For this review, take the finished solid that the model builds, in its own axes (mm). Face numbers are marked on the shaded views. A direction names the side the tool comes from. Give positions to 0.01 mm unless a question says otherwise; leave off trailing zeros. Loops run counter-clockwise (first coordinate to the right, second up) from the corner with the lowest first, then second, coordinate; pieces in that order, holes last.
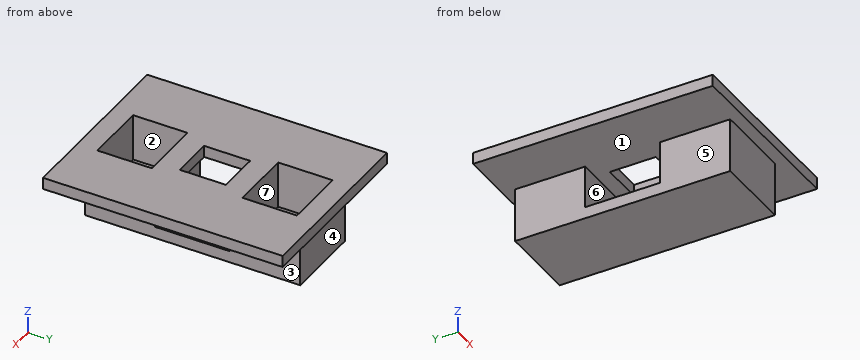
Autodesk Inventor part; units mm, degrees
ref_plane "Work Plane3" through (0, 0, 3.5) normal (0, 0, 1) x (1, 0, 0)
ref_plane "Work Plane2" through (0, 0, 0) normal (0, 0, -1) x (-1, 0, 0)
ref_plane "Work Plane1" through (0, 0, 0) normal (0, 0, -1) x (-1, 0, 0)
ref_plane "Work Plane3" through (0, 0, 3.5) normal (0, 0, 1) x (1, 0, 0)
sketch "Sketch2" plane through (0, 0, 3.5) normal (0, 0, 1) x (1, 0, 0)
  line L0 (-11.6713, -15.4051) -> (11.6713, -15.4051)
  line L1 (11.6713, -15.4051) -> (11.6713, 15.4051)
  line L2 (11.6713, 15.4051) -> (-11.6713, 15.4051)
  line L3 (-11.6713, 15.4051) -> (-11.6713, -15.4051)
  line L4 (-11.6713, -15.4051) -> (11.6713, 15.4051) construction
  line L5 (11.6713, -15.4051) -> (-11.6713, 15.4051) construction
  point P0 (0, 0)
  dimension "d4" = 30.8102
  dimension "d5" = 23.3426
extrude "Extrusion2" add sketch "Sketch2" along normal blind 1.5
ref_plane "Work Plane2" through (0, 0, 0) normal (0, 0, -1) x (-1, 0, 0)
sketch "Sketch3" plane through (0, 0, 0) normal (0, 0, -1) x (-1, 0, 0)
  line L0 (-2.7149, 2.9592) -> (2.7149, 2.9592)
  line L1 (2.7149, 2.9592) -> (2.7149, -2.9592)
  line L2 (2.7149, -2.9592) -> (-2.7149, -2.9592)
  line L3 (-2.7149, -2.9592) -> (-2.7149, 2.9592)
  line L4 (-2.7149, 2.9592) -> (2.7149, -2.9592) construction
  line L5 (2.7149, 2.9592) -> (-2.7149, -2.9592) construction
  point P0 (0, 0)
extrude "Extrusion3" cut sketch "Sketch3" against normal blind 6
ref_plane "Work Plane1" through (0, 0, 0) normal (0, 0, -1) x (-1, 0, 0)
sketch "Sketch4" plane through (0, 0, 0) normal (0, 0, -1) x (-1, 0, 0)
  line L0 (8.89, -12.7) -> (-8.89, -12.7)
  line L1 (3.6472, 12.7) -> (-3.3528, 12.7)
  line L2 (-3.3528, 12.7) -> (-3.3528, 7.7)
  line L3 (-3.3528, 7.7) -> (3.6472, 7.7)
  line L4 (3.6472, 7.7) -> (3.6472, 12.7)
  line L5 (3.6472, 12.7) -> (-3.3528, 7.7) construction
  line L6 (-3.3528, 12.7) -> (3.6472, 7.7) construction
  line L7 (-8.89, -12.7) -> (-8.89, 12.7)
  line L8 (3.6472, -7.7) -> (-3.3528, -7.7)
  line L9 (-3.3528, -7.7) -> (-3.3528, -12.7)
  line L10 (-3.3528, -12.7) -> (3.6472, -12.7)
  line L11 (3.6472, -12.7) -> (3.6472, -7.7)
  line L12 (3.6472, -7.7) -> (-3.3528, -12.7) construction
  line L13 (-3.3528, -7.7) -> (3.6472, -12.7) construction
  line L14 (-8.89, 12.7) -> (8.89, 12.7)
  point P0 (0, 0)
  point P1 (0.1472, 10.2)
  point P2 (0.1472, -10.2)
  point P3 (-3.3528, -10.2)
  dimension "d10" = 7
  dimension "d11" = 5
  dimension "d12" = 5.5372
  dimension "d13" = 7
  dimension "d14" = 5
  dimension "d15" = 5.5372
  dimension "d16" = 0
  dimension "d17" = 0
extrude "Extrusion4" cut sketch "Sketch4" against normal blind 3.5
sketch "Sketch5" plane through (0, 0, 3.5) normal (0, 0, -1) x (-1, 0, 0)
  line L0 (11.6713, -15.4051) -> (-11.6713, -15.4051)
  line L1 (-4.0005, -12.827) -> (3.9995, -12.827)
  line L2 (3.9995, -12.827) -> (3.9995, -5.827)
  line L3 (3.9995, -5.827) -> (-4.0005, -5.827)
  line L4 (-4.0005, -5.827) -> (-4.0005, -12.827)
  line L5 (-11.6713, -15.4051) -> (-11.6713, 15.4051)
  line L6 (2.7149, -2.9592) -> (-2.7149, -2.9592)
  line L7 (9.017, -12.827) -> (-9.017, -12.827)
  line L8 (-9.017, -12.827) -> (-9.017, 12.827)
  line L9 (-9.017, 12.827) -> (9.017, 12.827)
  line L10 (9.017, 12.827) -> (9.017, -12.827)
  line L11 (9.017, -12.827) -> (-9.017, 12.827) construction
  line L12 (-9.017, -12.827) -> (9.017, 12.827) construction
  line L13 (3.9995, 5.827) -> (-4.0005, 5.827)
  line L14 (-4.0005, 5.827) -> (-4.0005, 12.827)
  line L15 (-4.0005, 12.827) -> (3.9995, 12.827)
  line L16 (3.9995, 12.827) -> (3.9995, 5.827)
  line L17 (3.9995, 5.827) -> (-4.0005, 12.827) construction
  line L18 (-4.0005, 5.827) -> (3.9995, 12.827) construction
  line L19 (11.6713, 15.4051) -> (11.6713, -15.4051)
  point P0 (0, 0)
  point P1 (-0.0005, 9.327)
  point P2 (3.9995, 12.827)
  dimension "d20" = 8
  dimension "d21" = 7
  dimension "d22" = 7.6708
  dimension "d25" = 18.034
  dimension "d26" = 25.654
  dimension "d27" = 0
  dimension "d28" = 7
  dimension "d29" = 8
  dimension "d31" = 7.6718
extrude "Extrusion5" add sketch "Sketch5" along normal blind 4.5 contours L4 L3 L2 L1 | L9 L16 L13 L14
sketch "Sketch6" plane through (0, 0, -1) normal (0, 0, -1) x (-1, 0, 0)
  line L0 (4.9995, 13.827) -> (-5.0005, 13.827)
  line L1 (-5.0005, 13.827) -> (-5.0005, 4.827)
  line L2 (-5.0005, 4.827) -> (4.9995, 4.827)
  line L3 (4.9995, 4.827) -> (4.9995, 13.827)
  line L4 (4.9995, -4.827) -> (-5.0005, -4.827)
  line L5 (-5.0005, -4.827) -> (-5.0005, -13.827)
  line L6 (-5.0005, -13.827) -> (4.9995, -13.827)
  line L7 (4.9995, -13.827) -> (4.9995, -4.827)
  line L8 (-4.0005, 5.827) -> (3.9995, 5.827)
  line L9 (3.9995, 12.827) -> (-4.0005, 12.827)
  line L10 (3.9995, 5.827) -> (3.9995, 12.827)
  line L11 (-4.0005, 12.827) -> (-4.0005, 5.827)
  line L12 (-4.0005, -12.827) -> (3.9995, -12.827)
  line L13 (3.9995, -5.827) -> (-4.0005, -5.827)
  point P0 (0, 0)
  dimension "d35" = 1
  dimension "d36" = 1
  dimension "d37" = 1
  dimension "d38" = 1
  dimension "d39" = 1
  dimension "d40" = 1
extrude "Extrusion6" add sketch "Sketch6" along normal blind 1 and the other way blind 4.5 contours L3 L2 L1 L0 | L7 L6 L5 L4 | L11 L9 L10 L8
extrude "Extrusion7" cut sketch "Sketch5" along normal blind 4.5 and the other way blind 1.5 contours L4 L3 L2 L1 | L9 L16 L13 L14
sketch "Sketch8" plane through (0, 0, -2) normal (0, 0, -1) x (-1, 0, 0)
  line L0 (4.9995, 13.827) -> (4.9995, 4.827)
  line L1 (-5.0005, -13.827) -> (4.9995, -13.827)
  line L2 (4.9995, 13.827) -> (-5.0005, 13.827)
  line L3 (-5.0005, 13.827) -> (-5.0005, -13.827)
  line L4 (-5.0005, -13.827) -> (4.9995, -13.827)
  line L5 (4.9995, -13.827) -> (4.9995, 13.827)
  point P0 (0, 0)
extrude "Extrusion8" add sketch "Sketch8" along normal blind 1.5
properties part number "newairtempguytop"
Item 1: Clearance check with flat-ended pins moving along their axes: pin 1 Ø3 at (y, z) = (-10.5, 0.5) entering from +X; pin 2 Ø10 at (x, y) = (-6.5, 0.5) entering from -Z; pin 3 Ø4 at (y, z) = (11, -1.5) entering from -X; pin 4 Ø4.5 at (x, z) = (2, 1) entering from -Y. State where each tip first meets the part, or that it passes through.
Answer:
pin 1: stops at x = 5
pin 2: stops at z = -3.5
pin 3: stops at x = -5
pin 4: stops at y = -13.83
Item 2: Tool access review of the marked faces 4, 5, 6 and 7: name each direction out of +Z, -Z, +X, -X, +Y, -Y from which nothing blocks a thin tool from reaching the whole face with its end or side.
Answer:
face 4: -Z, +X, -X, +Y
face 5: -Z, -X, +Y, -Y
face 6: +X, -X
face 7: +Z
Item 3: Take a section at C-C on x = 4.5. Give the boundary of the cut face in (y, z).
Answer:
outline: (-15.41, 3.5) - (-13.83, 3.5) - (-13.83, -3.5) - (13.83, -3.5) - (13.83, 3.5) - (15.41, 3.5) - (15.41, 5) - (-15.41, 5) - close; hole (-4.83, -2) - (4.83, -2) - (4.83, 3.5) - (-4.83, 3.5) - close
Item 4: Take a section at A-A on z = 1.75. Give the boundary of the cut face in (x, y), and give its area (3 significant figures).
Answer:
outline: (-5, -13.83) - (5, -13.83) - (5, -4.83) - (-5, -4.83) - close; (-5, 4.83) - (5, 4.83) - (5, 13.83) - (-5, 13.83) - close; hole (-4, -12.83) - (4, -12.83) - (4, -5.83) - (-4, -5.83) - close; hole (-4, 5.83) - (4, 5.83) - (4, 12.83) - (-4, 12.83) - close
area: 68.0 mm2
Item 5: For L1, parallel to Y at x = -2.75, z = 4; L2, parallel to X at y = 7.5, z = 1.5; L3, parallel to Z at x = -1.5, y = -4, list the stretches that pass through material, from the lowest coordinate up.
Answer:
L1: y = -15.41 to -12.83, -5.83 to 5.83, 12.83 to 15.41
L2: x = -5 to -4, 4 to 5
L3: z = -3.5 to -2, 3.5 to 5
Item 6: Take a section at D-D on y = 13.5. Give the boundary of the cut face in (x, z).
Answer:
outline: (-11.67, 3.5) - (-5, 3.5) - (-5, -3.5) - (5, -3.5) - (5, 3.5) - (11.67, 3.5) - (11.67, 5) - (-11.67, 5) - close
Item 7: The part is to be moulded in two halves that separate along X. For the marked faces 1, 2 and 3, say which applies: released by +X, released by -X, zero draft, split by the parting line, or undercut.
Answer:
face 1: zero draft
face 2: undercut
face 3: released by +X
Item 8: Take a section at B-B on y = 4. Give the boundary of the cut face in (x, z).
Answer:
outline: (-11.67, 3.5) - (11.67, 3.5) - (11.67, 5) - (-11.67, 5) - close; (-5, -3.5) - (5, -3.5) - (5, -2) - (-5, -2) - close
